```python
from build123d import *

# Parameters (mm, degrees)
SKETCH1_R           = 10
SKETCH1_R_2         = 2.5
SKETCH1_W           = 7
SKETCH1_H           = 5
SKETCH1_W_2         = 5
SKETCH1_H_2         = 7
BOSS_EXTRUDE1_DEPTH = 1
FILLET1_R           = 10
CUT_EXTRUDE3_DEPTH  = 362.864615568
SKETCH6_W           = 10
SKETCH6_H           = 12
CUT_EXTRUDE5_DEPTH  = 10
SKETCH7_W           = 6
SKETCH7_H           = 7
CUT_EXTRUDE6_DEPTH  = 362.864615568
SKETCH3_R           = 1.25
CUT_EXTRUDE2_DEPTH  = 362.864615568
FILLET2_R           = 0.5


with BuildPart() as part:
    # Sketch1 → Boss-Extrude1 (new body)
    with BuildSketch(Plane(origin=(0, 0, 0), x_dir=(1, 0, 0), z_dir=(0, 1, 0))):
        Polygon((77, 0), (77, 175), (253, 175), (253, 0), (281, 0), (281, 228), (0, 228), (0, 0), align=None)
        with Locations(Location((24.25, 104.25, 0), (0, 0, 270))):
            Circle(SKETCH1_R, mode=Mode.SUBTRACT)
        with Locations(Location((6, 222, 0), (0, 0, 270))):
            Circle(SKETCH1_R_2, mode=Mode.SUBTRACT)
        with Locations(Location((6, 5, 0), (0, 0, 270))):
            Circle(SKETCH1_R_2, mode=Mode.SUBTRACT)
        with Locations(Location((275, 222, 0), (0, 0, 270))):
            Circle(SKETCH1_R_2, mode=Mode.SUBTRACT)
        with Locations((273, 7.5)):
            Rectangle(SKETCH1_W, SKETCH1_H, mode=Mode.SUBTRACT)
        with Locations((272.5, 170)):
            Rectangle(SKETCH1_W_2, SKETCH1_H_2, mode=Mode.SUBTRACT)
        with Locations((64.5, 7.5)):
            Rectangle(SKETCH1_W, SKETCH1_H, mode=Mode.SUBTRACT)
        with Locations((66, 167.5)):
            Rectangle(SKETCH1_W, SKETCH1_H, mode=Mode.SUBTRACT)
    extrude(amount=BOSS_EXTRUDE1_DEPTH)

    # Fillet1
    fillet1_edges = [part.edges().sort_by_distance(p)[0] for p in [
        (253, 0.5, -175),
        (77, 0.5, -175),
    ]]
    fillet(fillet1_edges, radius=FILLET1_R)

    # Sketch4 → Cut-Extrude3 (cut, through all)
    with BuildSketch(Plane(origin=(0, 1, 0), x_dir=(1, 0, 0), z_dir=(0, 1, 0))):
        with BuildLine():
            Line((53.5, 212.5), (53.5, 193.5))
            ThreePointArc((53.5, 193.5), (51, 191), (48.5, 193.5))
            Line((48.5, 193.5), (48.5, 212.5))
            ThreePointArc((48.5, 212.5), (51, 215), (53.5, 212.5))
        make_face()
        with BuildLine():
            Line((43.5, 212.5), (43.5, 193.5))
            ThreePointArc((43.5, 193.5), (41, 191), (38.5, 193.5))
            Line((38.5, 193.5), (38.5, 212.5))
            ThreePointArc((38.5, 212.5), (41, 215), (43.5, 212.5))
        make_face()
        with BuildLine():
            Line((33.5, 212.5), (33.5, 193.5))
            ThreePointArc((33.5, 193.5), (31, 191), (28.5, 193.5))
            Line((28.5, 193.5), (28.5, 212.5))
            ThreePointArc((28.5, 212.5), (31, 215), (33.5, 212.5))
        make_face()
        with BuildLine():
            Line((23.5, 212.5), (23.5, 193.5))
            ThreePointArc((23.5, 193.5), (21, 191), (18.5, 193.5))
            Line((18.5, 193.5), (18.5, 212.5))
            ThreePointArc((18.5, 212.5), (21, 215), (23.5, 212.5))
        make_face()
        with BuildLine():
            Line((13.5, 212.5), (13.5, 193.5))
            ThreePointArc((13.5, 193.5), (11, 191), (8.5, 193.5))
            Line((8.5, 193.5), (8.5, 212.5))
            ThreePointArc((8.5, 212.5), (11, 215), (13.5, 212.5))
        make_face()
    extrude(amount=-CUT_EXTRUDE3_DEPTH, mode=Mode.SUBTRACT)

    # Sketch6 → Cut-Extrude5 (cut)
    with BuildSketch(Plane(origin=(0, 1, 0), x_dir=(1, 0, 0), z_dir=(0, 1, 0))):
        with Locations((105.19, 185.6)):
            Rectangle(SKETCH6_W, SKETCH6_H)
    extrude(amount=-CUT_EXTRUDE5_DEPTH, mode=Mode.SUBTRACT)

    # Sketch7 → Cut-Extrude6 (cut, through all)
    with BuildSketch(Plane(origin=(0, 1, 0), x_dir=(1, 0, 0), z_dir=(0, 1, 0))):
        with Locations((92.74, 186.1)):
            Rectangle(SKETCH7_W, SKETCH7_H)
    extrude(amount=-CUT_EXTRUDE6_DEPTH, mode=Mode.SUBTRACT)

    # Sketch3 → Cut-Extrude2 (cut, through all)
    with BuildSketch(Plane(origin=(0, 1, 0), x_dir=(1, 0, 0), z_dir=(0, 1, 0))):
        with Locations((275.616116524, 5.883883476)):
            Circle(SKETCH3_R)
        with Locations((275.616116524, 9.116116524)):
            Circle(SKETCH3_R)
        with Locations((270.383883476, 9.116116524)):
            Circle(SKETCH3_R)
        with Locations((270.383883476, 5.883883476)):
            Circle(SKETCH3_R)
        with Locations((274.116116524, 167.383883476)):
            Circle(SKETCH3_R)
        with Locations((270.883883476, 167.383883476)):
            Circle(SKETCH3_R)
        with Locations((274.116116524, 172.616116524)):
            Circle(SKETCH3_R)
        with Locations((270.883883476, 172.616116524)):
            Circle(SKETCH3_R)
        with Locations((67.116116524, 9.116116524)):
            Circle(SKETCH3_R)
        with Locations((67.116116524, 5.883883476)):
            Circle(SKETCH3_R)
        with Locations((61.883883476, 5.883883476)):
            Circle(SKETCH3_R)
        with Locations((61.883883476, 9.116116524)):
            Circle(SKETCH3_R)
        with Locations((63.383883476, 165.883883476)):
            Circle(SKETCH3_R)
        with Locations((63.383883476, 169.116116524)):
            Circle(SKETCH3_R)
        with Locations((68.616116524, 169.116116524)):
            Circle(SKETCH3_R)
        with Locations((68.616116524, 165.883883476)):
            Circle(SKETCH3_R)
        with Locations((90.62, 188.72)):
            Circle(SKETCH3_R)
        with Locations((94.86, 188.72)):
            Circle(SKETCH3_R)
        with Locations((90.62, 183.48)):
            Circle(SKETCH3_R)
        with Locations((94.86, 183.48)):
            Circle(SKETCH3_R)
        with Locations((101.073883476, 190.716116524)):
            Circle(SKETCH3_R)
        with Locations((109.306116524, 180.483883476)):
            Circle(SKETCH3_R)
        with Locations((109.306116524, 190.716116524)):
            Circle(SKETCH3_R)
        with Locations((101.073883476, 180.483883476)):
            Circle(SKETCH3_R)
    extrude(amount=-CUT_EXTRUDE2_DEPTH, mode=Mode.SUBTRACT)

    # Fillet2
    fillet2_edges = [part.edges().sort_by_distance(p)[0] for p in [
        (0, 0.5, 0),
        (0, 0.5, -228),
        (281, 0.5, -228),
        (281, 0.5, 0),
        (253, 0.5, 0),
        (77, 0.5, 0),
    ]]
    fillet(fillet2_edges, radius=FILLET2_R)


solid = part.part
```
Here's how the part is built. I have some questions about the finished solid (model axes, mm). Coordinates: 2 decimals unless noted, no trailing zeros. Loops run counter-clockwise (first coordinate to the right, second up) from the corner with the lowest first, then second, coordinate; pieces in that order, holes last. Notation, with made-up numbers: (65, -11.75) - (115, -11.75) arc R16 ccw to (115, 5.25) - close; hole circle Ø1 at (60, 41). An arc over 180 degrees is marked (long way). Answer as CSV lines item,"result".
Q1. If I drill on L1, parallel to X at y = 0.65, z = -222; L2, parallel to X at y = 0.8, z = -104.25; L3, parallel to X at y = 0.4, z = -130.5, over which ranges is the centre line in solid material (lowest first)? Write a range as [from, to].
Response:
L1,"[0, 3.5], [8.5, 272.5], [277.5, 281]"
L2,"[0, 14.25], [34.25, 77], [253, 281]"
L3,"[0, 77], [253, 281]"
Q2. If we section it at A-A, the plane z = -40: Write out the boundary of the cut face in (x, y).
Response:
outline,"(0, 0) - (77, 0) - (77, 1) - (0, 1) - close; (253, 0) - (281, 0) - (281, 1) - (253, 1) - close"
Q3. If we section it at C-C, the plane y = 0.85: Give the number of separate pieces and of enclosed holes in the cut face, and give its area (3 significant figures).
Response:
separate pieces,"1"
enclosed holes,"15"
area,"32,000 mm2"
Q4. If we section it at B-B, the plane x = 171: Write out the boundary of the cut face in (y, z).
Response:
outline,"(0, -228) - (1, -228) - (1, -175) - (0, -175) - close"
Q5. We'd pull the mould along X, two halves only. Please class faces 1 (the face through (79.85, 0.51, -171.99)), 2 (the face through (249.99, 0.51, -172.15)), 3 (the face through (76, 1, -141)): pulls with the +X half, pulls with the -X half, needs draft (parallel to the pull), parting line crosses it, or undercut.
Response:
face 1,"undercut"
face 2,"undercut"
face 3,"needs draft"
